Autodesk Inventor part; units mm, degrees
ref_plane "MSC_PT1" through (0, 0, 3.2) normal (0, 0, 1) x (1, 0, 0)
ref_plane "MSC_PT2" through (0, 0, 0) normal (0, 0, -1) x (-1, 0, 0)
ref_plane "MSC_PF1" through (0, 0, 0) normal (1, 0, 0) x (0, 1, 0)
sketch "Sketch1" plane through (0, 0, 0) normal (0, 0, 1) x (1, 0, 0)
  circle A0 centre (0, 0) radius 5 construction
  line L0 (-5, 2.8868) -> (-5, -2.8868)
  line L1 (-5, -2.8868) -> (0, -5.7735)
  line L2 (0, -5.7735) -> (5, -2.8868)
  line L3 (5, -2.8868) -> (5, 2.8868)
  line L4 (5, 2.8868) -> (0, 5.7735)
  line L5 (0, 5.7735) -> (-5, 2.8868)
  line L6 (0, 8.0829) -> (0, -8.0829)
  line L7 (-7, 0) -> (7, 0)
  point P0 (0, 0)
  dimension "ParS" = 10
extrude "Extrusion1" add sketch "Sketch1" along normal blind 3.2
sketch "Sketch2" plane through (0, 0, 3.2) normal (0, 0, 1) x (1, 0, 0)
  point P0 (0, 0)
  point P1 (0, 0)
hole "Hole1" at (0, 0, 3.2) direction (0, 0, -1) diameter 4.917 end through all
ref_plane "MSC_PT1" through (0, 0, 3.2) normal (0, 0, 1) x (1, 0, 0)
ref_plane "MSC_PT2" through (0, 0, 0) normal (0, 0, -1) x (-1, 0, 0)
ref_plane "MSC_PF1" through (0, 0, 0) normal (1, 0, 0) x (0, 1, 0)
chamfer "Chamfer1" distance 0.6 angle 45 2 edges at (0, 2.4585, 3.2) (0, 2.4585, 0)
equation "\"d17\" = 0.6 * PTC"
equation "\"d18\" = 0.6 * PTC"
equation "\"d4\" = M"
equation "\"PTC\" = 1"
equation "\"NND\" = 6"
equation "\"THREADDIA\" = NND"
properties part number "ISO 4036 - M6" material "Steel"
Source: CAD feature listing. Evaluate the final solid. Frame: model axes, mm. Coordinates: 2 decimals unless noted, no trailing zeros. Order: outer loops, then holes, each group sorted by start corner. A loop starts at its lowest first (then second) coordinate and runs counter-clockwise, first axis right, second up. Notation, with made-up numbers: M 44,-35.5 L 50,-35.5 A33 ccw 50,0.5 Z; hole C 7,-11 d5. An arc over 180 degrees is marked long. Write each question's results on one line, items separated by ' | '. Start each with the question number.
Item 1: Cut plane B-B (z = 1). Return loops of the section in (x, y), and give its area (3 significant figures).
Item 2: Line query: probe 1 along X at (y, z) = (0, 2.2); probe 2 along X at (y, z) = (-1.5, 1.95); probe 3 along Y at (x, z) = (-1.25, 1.45). Output: solid intervals per line, ascending.
Item 3: Cut plane C-C (y = -4.25). Return loops of the section in (x, z).
Item 4: Cut plane D-D (y = 5). Return loops of the section in (x, z), and give its area (3 significant figures).
Item 5: Draft query along Y for faces 1 (the face through (-2.535, -4.31, 1.578)), 2 (the face through (-0.738, -2.345, 1.586)), 3 (the face through (-2.465, 4.35, 1.578)). Return one class per face: pulls with the +Y half, pulls with the -Y half, needs draft (parallel to the pull), parting line crosses it, or undercut.
Item 6: Cut plane A-A (y = 0). Return loops of the section in (x, z).
Item 7: First-contact query: pin 1 Ø3 at (x, y) = (4, 2.5) entering from -Z; pin 2 Ø5.5 at (x, y) = (0, 0) entering from +Z. Flat tips, straight axial feed; report the tip coordinate or a pass-through.
Checked values:
1) outline: M -5,-2.89 L 0,-5.77 L 5,-2.89 L 5,2.89 L 0,5.77 L -5,2.89 Z; hole C 0,0 d4.92 | area: 67.6 mm2
2) probe 1: x = -5 to -2.46, 2.46 to 5 | probe 2: x = -5 to -1.95, 1.95 to 5 | probe 3: y = -5.05 to -2.12, 2.12 to 5.05
3) outline: M -2.64,0 L 2.64,0 L 2.64,3.2 L -2.64,3.2 Z
4) outline: M -1.34,0 L 1.34,0 L 1.34,3.2 L -1.34,3.2 Z | area: 8.57 mm2
5) face 1: pulls with the -Y half | face 2: undercut | face 3: pulls with the +Y half
6) outline: M -5,0 L -3.06,0 L -2.46,0.6 L -2.46,2.6 L -3.06,3.2 L -5,3.2 Z; M 2.46,0.6 L 3.06,0 L 5,0 L 5,3.2 L 3.06,3.2 L 2.46,2.6 Z
7) pin 1: stops at z = 0 | pin 2: stops at z = 2.89
